from build123d import *

# Parameters (mm, degrees)
F0_R     = 30
F1_DEPTH = 197.5
F2_DEPTH = 98.75
F5_R     = 30
F6_DEPTH = 197.5


with BuildPart() as f1:
    # F0 (on Front) → F1 (new body, symmetric)
    with BuildSketch(Plane.XZ):
        Circle(F0_R)
    extrude(amount=F1_DEPTH, both=True)



with BuildPart() as f2:
    # F0 (on Front) → F2 (new body, symmetric)
    with BuildSketch(Plane.XZ):
        with Locations((197.5, 0)):
            Circle(F0_R)
    extrude(amount=F2_DEPTH, both=True)


with BuildPart() as f4_1:
    # F4: instance of F1
    add(f1.part.mirror(Plane.YZ.offset(197.5)))


with BuildPart() as f1_1:
    add(f1.part)

    add(f2.part)  # F6 merges F2

    add(f4_1.part)  # F6 merges F4_1
    # F5 (on plane+point) → F6 (join, symmetric)
    with BuildSketch(Plane.YZ.offset(197.5)):
        with Locations((-98.75, 0)):
            Circle(F5_R)
        with Locations((98.75, 0)):
            Circle(F5_R)
    extrude(amount=F6_DEPTH, both=True)


solid = f1_1.part
Geometry check sheet. Reference: the model listing, model coordinates, mm. A direction names the side the tool comes from. Round coordinates to 2 decimals unless told otherwise and drop trailing zeros. Loops run counter-clockwise (first coordinate to the right, second up) from the corner with the lowest first, then second, coordinate; pieces in that order, holes last. Notation, with made-up numbers: (7.5, 61.25) - (49.5, 61.25) arc R6 cw to (49.5, 65.25) - close; hole circle Ø11 at (87, -33.75). An arc over 180 degrees is marked (long way). Answer as CSV lines item,"result".
(1) Cross-section at A-A, the plane y = 28.5. Enter the section's corners in (x, z).
Output values:
outline,"circle Ø60 at (0, 0); circle Ø60 at (197.5, 0); circle Ø60 at (395, 0)"
(2) Cross-section at B-B, the plane x = 331. Enter the section's corners in (y, z), and give its area (3 significant figures).
Output values:
outline,"circle Ø60 at (-98.75, 0); circle Ø60 at (98.75, 0)"
area,"5,650 mm²"
(3) Set-up check for faces 1 (the face through (0, 197.5, 0)), 2 (the face through (167.53, -1.38, 1.32)): record each of +Z, -Z, +X, -X, +Y, -Y from which the full face is reachable in a straight line by a thin tool's end or side.
Output values:
face 1,"+Z, -Z, +X, -X, +Y"
face 2,"none"
(4) Cross-section at C-C, the plane z = -21.5. Enter the section's corners in (x, y).
Output values:
outline,"(-20.92, -197.5) - (20.92, -197.5) - (20.92, -119.67) - (374.08, -119.67) - (374.08, -197.5) - (415.92, -197.5) - (415.92, 197.5) - (374.08, 197.5) - (374.08, 119.67) - (20.92, 119.67) - (20.92, 197.5) - (-20.92, 197.5) - close; hole (20.92, -77.83) - (176.58, -77.83) - (176.58, 77.83) - (20.92, 77.83) - close; hole (218.42, -77.83) - (374.08, -77.83) - (374.08, 77.83) - (218.42, 77.83) - close"
(5) Depth check by flat-ended pin: pin 1 Ø5 at (x, z) = (315.5, 11.5) entering from -Y; pin 2 Ø6 at (y, z) = (85.5, -19.5) entering from -X; pin 3 Ø10 at (x, z) = (190.5, -12.5) entering from +Y. Enter the tip coordinate at first touch or a pass-through.
Output values:
pin 1,"stops at y = -127.37"
pin 2,"stops at x = -25.05"
pin 3,"stops at y = 127.8"
(6) Material ranges on line 1 along X through (y, z) = (46, -17); line 2 along Y through (x, z) = (36.5, 13); line 3 along Y through (x, z) = (79.5, 16), recorded low to high.
Output values:
line 1,"x = -24.72 to 24.72, 172.78 to 222.22, 370.28 to 419.72"
line 2,"y = -125.79 to -71.71, 71.71 to 125.79"
line 3,"y = -124.13 to -73.37, 73.37 to 124.13"
(7) Cross-section at D-D, the plane y = 143.5. Enter the section's corners in (x, z).
Output values:
outline,"circle Ø60 at (0, 0); circle Ø60 at (395, 0)"
